from build123d import *

# Parameters (mm, degrees)
SKETCH_1_W          = 85
SKETCH_1_H          = 100
EXTRUDE_1_DEPTH     = 3
SKETCH_2_W          = 3
SKETCH_2_H          = 100
EXTRUDE_2_DEPTH     = 30
CUT_EXTRUDE_1_REACH = 105.99
SKETCH_3_R          = 4
SKETCH_4_R          = 3
SKETCH_4_R_2        = 2
SKETCH_4_R_3        = 2.445405454
CUT_EXTRUDE_3_DEPTH = 74.452365517


with BuildPart() as part:
    # 草图1 → 凸台-拉伸1 (new body)
    with BuildSketch(Plane(origin=(0, 0, 0), x_dir=(1, 0, 0), z_dir=(0, 1, 0))):
        Rectangle(SKETCH_1_W, SKETCH_1_H)
    extrude(amount=EXTRUDE_1_DEPTH)

    # 草图2 → 凸台-拉伸2 (add)
    with BuildSketch(Plane(origin=(0, 3, 0), x_dir=(1, 0, 0), z_dir=(0, 1, 0))):
        with Locations((-41, 0)):
            Rectangle(SKETCH_2_W, SKETCH_2_H)
        with Locations((41, 0)):
            Rectangle(SKETCH_2_W, SKETCH_2_H)
    extrude(amount=EXTRUDE_2_DEPTH)

    # 切除-拉伸1: up to this face of the body (flat: up to its plane)
    cut_extrude_1_end = Plane(part.part.faces().sort_by_distance((-42.5, 16.5, 0))[0])
    # 草图3 → 切除-拉伸1 (cut, up to the picked face)
    with BuildSketch(Plane(origin=(42.5, 0, 0), x_dir=(0, 0, -1), z_dir=(1, 0, 0)), mode=Mode.PRIVATE) as cut_extrude_1_sk1:
        with Locations((42.5, 16.5)):
            Circle(SKETCH_3_R)
    cut_extrude_1_tool1 = split(extrude(cut_extrude_1_sk1.sketch, amount=-CUT_EXTRUDE_1_REACH, mode=Mode.PRIVATE), bisect_by=cut_extrude_1_end, keep=Keep.BOTH, mode=Mode.PRIVATE)
    # 草图3 → 切除-拉伸1 (cut, up to the picked face)
    with BuildSketch(Plane(origin=(42.5, 0, 0), x_dir=(0, 0, -1), z_dir=(1, 0, 0)), mode=Mode.PRIVATE) as cut_extrude_1_sk2:
        with BuildLine():
            Line((-42.5, 12.5), (17.5, 12.5))
            ThreePointArc((17.5, 12.5), (21.5, 16.5), (17.5, 20.5))
            Line((17.5, 20.5), (-42.5, 20.5))
            ThreePointArc((-42.5, 20.5), (-46.5, 16.5), (-42.5, 12.5))
        make_face()
    cut_extrude_1_tool2 = split(extrude(cut_extrude_1_sk2.sketch, amount=-CUT_EXTRUDE_1_REACH, mode=Mode.PRIVATE), bisect_by=cut_extrude_1_end, keep=Keep.BOTH, mode=Mode.PRIVATE)
    add(cut_extrude_1_tool1.solids().sort_by(Axis((42.5, 16.5, -42.5), (-1, 0, 0)))[0], mode=Mode.SUBTRACT)
    add(cut_extrude_1_tool2.solids().sort_by(Axis((42.5, 16.5, 12.5), (-1, 0, 0)))[0], mode=Mode.SUBTRACT)

    # 草图4 → 切除-拉伸3 (cut, through all)
    with BuildSketch(Plane.XZ):
        with Locations(Location((21, 0, 0), (0, 0, 270))):
            Circle(SKETCH_4_R)
        with Locations(Location((10, -22.5, 0), (0, 0, 270))):
            Circle(SKETCH_4_R)
        with Locations(Location((32, -22.5, 0), (0, 0, 270))):
            Circle(SKETCH_4_R)
        with Locations(Location((10, 22.5, 0), (0, 0, 270))):
            Circle(SKETCH_4_R)
        with Locations(Location((32, 22.5, 0), (0, 0, 270))):
            Circle(SKETCH_4_R)
        with Locations(Location((21, -45, 0), (0, 0, 270))):
            Circle(SKETCH_4_R_2)
        with Locations(Location((-34, 15, 0), (0, 0, 270))):
            Circle(SKETCH_4_R_3)
    extrude(amount=-CUT_EXTRUDE_3_DEPTH, mode=Mode.SUBTRACT)


solid = part.part
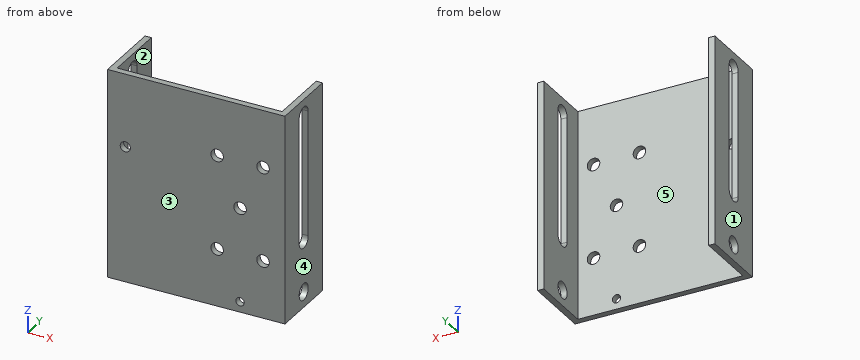
The model under review builds one solid part; all positions refer to its coordinate system, in mm. Face numbers are marked on the shaded views. A direction names the side the tool comes from. Coordinates: 2 decimals unless noted, no trailing zeros. Loops run counter-clockwise (first coordinate to the right, second up) from the corner with the lowest first, then second, coordinate; pieces in that order, holes last.
(1) Consider section C-C, the plane y = 7.5. Give the boundary of the cut face in (x, z), plus the area to 3 significant figures.
Determined:
outline: (-42.5, -50) - (-39.5, -50) - (-39.5, 50) - (-42.5, 50) - close; (39.5, -50) - (42.5, -50) - (42.5, 50) - (39.5, 50) - close
area: 600 mm2
(2) Wall thickness on L1, parallel to X at y = 8.5, z = -36; L2, parallel to X at y = 1.8, z = -45; L3, parallel to Z at x = 41, y = 16: over which ranges is each line inside the solid? List them lowest first.
Determined:
L1: x = -42.5 to -39.5, 39.5 to 42.5
L2: x = -42.5 to 19, 23 to 42.5
L3: z = -50 to -46.47, -38.53 to -21.47, 46.47 to 50
(3) Consider section D-D, the plane z = -15.5. Give the boundary of the cut face in (x, y).
Determined:
outline: (-42.5, 0) - (42.5, 0) - (42.5, 12.5) - (39.5, 12.5) - (39.5, 3) - (-39.5, 3) - (-39.5, 12.5) - (-42.5, 12.5) - close; (-42.5, 20.5) - (-39.5, 20.5) - (-39.5, 33) - (-42.5, 33) - close; (39.5, 20.5) - (42.5, 20.5) - (42.5, 33) - (39.5, 33) - close
(4) Draft analysis for pull direction X (two halves, no side actions). For the marked faces 3, 4 and 5, state which applies: +X half, -X half, draft (parallel to the pull), parting line (faces both ways), or undercut.
Determined:
face 3: draft
face 4: +X half
face 5: undercut
(5) Consider section A-A, the plane z = 22.5. Give the boundary of the cut face in (x, y), plus the area to 3 significant figures.
Determined:
outline: (-42.5, 0) - (7, 0) - (7, 3) - (-39.5, 3) - (-39.5, 12.5) - (-42.5, 12.5) - close; (-42.5, 20.5) - (-39.5, 20.5) - (-39.5, 33) - (-42.5, 33) - close; (13, 0) - (29, 0) - (29, 3) - (13, 3) - close; (35, 0) - (42.5, 0) - (42.5, 12.5) - (39.5, 12.5) - (39.5, 3) - (35, 3) - close; (39.5, 20.5) - (42.5, 20.5) - (42.5, 33) - (39.5, 33) - close
area: 351 mm2
(6) Tool access review of the marked faces 1 and 2: name each direction out of +Z, -Z, +X, -X, +Y, -Y from which nothing blocks a thin tool from reaching the whole face with its end or side.
Determined:
face 1: +Z, -Z, -X, +Y, -Y
face 2: +Z, -Z, +Y
(7) Insertion check: P1, Ø8, axis at x = 10, z = -22.5, coming from the +Y side. The pin has a flat end and moves straight along its axis. Give the tip position at first contact, or say it passes through.
Determined:
P1: stops at y = 3
(8) Consider section B-B, the plane x = 32. Give the boundary of the cut face in (y, z).
Determined:
outline: (0, -50) - (3, -50) - (3, -25.5) - (0, -25.5) - close; (0, -19.5) - (3, -19.5) - (3, 19.5) - (0, 19.5) - close; (0, 25.5) - (3, 25.5) - (3, 50) - (0, 50) - close
